Autodesk Inventor part; units mm, degrees
ref_plane "YZ Plane" through (0, 0, 0) normal (1, 0, 0) x (0, 1, 0)
ref_plane "XZ Plane" through (0, 0, 0) normal (0, 1, 0) x (-1, 0, 0)
ref_plane "XY Plane" through (0, 0, 0) normal (0, 0, 1) x (1, 0, 0)
sketch "CONTOURS" plane through (0, 0, 0) normal (0, 0, 1) x (1, 0, 0)
  line L0 (2153.8888, 619.2359) -> (2163.4719, 633.117)
  arc A0 (2185.9832, 634.7957) -> (2163.4719, 633.117) centre (2175.4045, 624.8791) ccw
  line L1 (2185.9832, 634.7957) -> (2411.1355, 394.6117)
  arc A1 (2406.7717, 371.5944) -> (2411.1355, 394.6117) centre (2400.5567, 384.695) ccw
  line L2 (2406.7717, 371.5944) -> (2360.367, 349.5799)
  arc A2 (2360.367, 349.5799) -> (2354.7432, 326.1016) centre (2367.0105, 335.5759) ccw
  line L3 (2354.7432, 326.1016) -> (2420.766, 240.6152)
  arc A3 (991.9076, 405.3519) -> (2420.766, 240.6152) centre (1790.9625, 1056.9921) ccw
  line L4 (991.9076, 405.3519) -> (1516.221, 700.5434)
  arc A4 (1516.221, 700.5434) -> (2065.5544, 700.5434) centre (1790.8877, 1057.1243) ccw
  line L5 (2065.5544, 700.5434) -> (2128.8659, 618.5677)
  arc A5 (2128.8659, 618.5677) -> (2153.8888, 619.2359) centre (2141.1332, 628.042) ccw
sketch "HOLES" plane through (0, 0, 0) normal (0, 0, 1) x (1, 0, 0)
  arc A0 (1449.9335, 932.975) -> (1455.5442, 933.6958) centre (1452.3785, 936.1408) ccw
  line L0 (1449.9335, 932.975) -> (1421.4416, 954.9799)
  arc A1 (1420.7208, 960.5906) -> (1421.4416, 954.9799) centre (1423.8866, 958.1456) ccw
  line L1 (1420.7208, 960.5906) -> (1427.4445, 969.2965)
  arc A2 (1433.0553, 970.0172) -> (1427.4445, 969.2965) centre (1430.6103, 966.8515) ccw
  line L2 (1433.0553, 970.0172) -> (1461.5471, 948.0124)
  arc A3 (1462.2679, 942.4017) -> (1461.5471, 948.0124) centre (1459.1022, 944.8467) ccw
  line L3 (581.1233, 599.0223) -> (574.9213, 608.1072)
  arc A4 (574.9213, 608.1072) -> (569.3624, 609.1555) centre (571.6177, 605.8519) ccw
  line L4 (569.3624, 609.1555) -> (539.6301, 588.858)
  arc A5 (539.6301, 588.858) -> (538.5818, 583.2991) centre (541.8854, 585.5544) ccw
  line L5 (538.5818, 583.2991) -> (544.7838, 574.2142)
  arc A6 (544.7838, 574.2142) -> (550.3427, 573.1659) centre (548.0874, 576.4695) ccw
  line L6 (550.3427, 573.1659) -> (580.075, 593.4634)
  arc A7 (580.075, 593.4634) -> (581.1233, 599.0223) centre (577.8197, 596.767) ccw
  line L7 (1171.3736, 565.7512) -> (1178.0973, 574.4571)
  arc A8 (1178.0973, 574.4571) -> (1177.3765, 580.0678) centre (1174.9316, 576.9021) ccw
  line L8 (1177.3765, 580.0678) -> (1148.8847, 602.0727)
  arc A9 (1148.8847, 602.0727) -> (1143.2739, 601.3519) centre (1146.4397, 598.9069) ccw
  line L9 (1143.2739, 601.3519) -> (1136.5502, 592.646)
  arc A10 (1136.5502, 592.646) -> (1137.271, 587.0353) centre (1139.716, 590.201) ccw
  line L10 (1137.271, 587.0353) -> (1165.7629, 565.0304)
  arc A11 (1165.7629, 565.0304) -> (1171.3736, 565.7512) centre (1168.2079, 568.1962) ccw
  line L11 (312.7987, 992.0706) -> (319.0007, 982.9857)
  arc A12 (317.9524, 977.4269) -> (319.0007, 982.9857) centre (315.6972, 980.7305) ccw
  line L12 (317.9524, 977.4269) -> (288.2201, 957.1293)
  arc A13 (282.6613, 958.1776) -> (288.2201, 957.1293) centre (285.9648, 960.4329) ccw
  line L13 (282.6613, 958.1776) -> (276.4592, 967.2625)
  arc A14 (277.5075, 972.8214) -> (276.4592, 967.2625) centre (279.7628, 969.5178) ccw
  line L14 (277.5075, 972.8214) -> (307.2399, 993.1189)
  arc A15 (312.7987, 992.0706) -> (307.2399, 993.1189) centre (309.4951, 989.8153) ccw
  arc A16 (877.4586, 807.9096) -> (881.5741, 811.7907) centre (877.5758, 811.9079) ccw
  line L15 (881.5741, 811.7907) -> (887.6999, 1020.7009)
  arc A17 (887.6999, 1020.7009) -> (883.8189, 1024.8164) centre (883.7016, 1020.8181) ccw
  line L16 (883.8189, 1024.8164) -> (872.8236, 1025.1388)
  arc A18 (872.8236, 1025.1388) -> (868.7081, 1021.2578) centre (872.7064, 1021.1405) ccw
  line L17 (868.7081, 1021.2578) -> (862.5822, 812.3476)
  arc A19 (862.5822, 812.3476) -> (866.4633, 808.232) centre (866.5805, 812.2303) ccw
  line L18 (866.4633, 808.232) -> (877.4586, 807.9096)
  arc A20 (370.076, 874.2818) -> (369.0277, 868.7229) centre (372.3312, 870.9782) ccw
  line L19 (369.0277, 868.7229) -> (486.8661, 696.1104)
  arc A21 (486.8661, 696.1104) -> (492.425, 695.062) centre (490.1697, 698.3656) ccw
  line L20 (492.425, 695.062) -> (501.5098, 701.2641)
  arc A22 (501.5098, 701.2641) -> (502.5581, 706.8229) centre (499.2546, 704.5677) ccw
  line L21 (502.5581, 706.8229) -> (384.7197, 879.4355)
  arc A23 (384.7197, 879.4355) -> (379.1608, 880.4838) centre (381.4161, 877.1802) ccw
  line L22 (379.1608, 880.4838) -> (370.076, 874.2818)
  line L23 (1833.6661, 426.4523) -> (1844.634, 427.2924)
  arc A24 (1833.6661, 426.4523) -> (1829.9832, 422.1586) centre (1833.9716, 422.464) ccw
  line L24 (1845.9439, 213.7689) -> (1829.9832, 422.1586)
  arc A25 (1101.2975, 659.9143) -> (1095.6868, 659.1936) centre (1098.8525, 656.7486) ccw
  arc A26 (1845.9439, 213.7689) -> (1850.2377, 210.086) centre (1849.9322, 214.0744) ccw
  arc A27 (2077.5111, 618.774) -> (2071.8727, 619.2297) centre (2074.4641, 616.1826) ccw
  line L25 (620.0838, 641.0058) -> (644.8608, 657.9204)
  arc A28 (644.8608, 657.9204) -> (645.9091, 663.4793) centre (642.6055, 661.224) ccw
  line L26 (645.9091, 663.4793) -> (639.707, 672.5642)
  arc A29 (639.707, 672.5642) -> (634.1482, 673.6125) centre (636.4035, 670.3089) ccw
  line L27 (634.1482, 673.6125) -> (609.3712, 656.6979)
  arc A30 (609.3712, 656.6979) -> (608.3229, 651.139) centre (611.6265, 653.3943) ccw
  line L28 (608.3229, 651.139) -> (614.525, 642.0541)
  arc A31 (614.525, 642.0541) -> (620.0838, 641.0058) centre (617.8286, 644.3094) ccw
  line L29 (1089.6839, 644.877) -> (1113.4271, 626.5396)
  arc A32 (1113.4271, 626.5396) -> (1119.0379, 627.2604) centre (1115.8721, 629.7054) ccw
  line L30 (1119.0379, 627.2604) -> (1125.7616, 635.9662)
  arc A33 (1125.7616, 635.9662) -> (1125.0408, 641.577) centre (1122.5958, 638.4112) ccw
  line L31 (1125.0408, 641.577) -> (1101.2975, 659.9143)
  arc A34 (1553.2327, 613.0929) -> (1551.9237, 618.5962) centre (1549.8265, 615.19) ccw
  line L32 (1095.6868, 659.1936) -> (1088.9631, 650.4877)
  arc A35 (1088.9631, 650.4877) -> (1089.6839, 644.877) centre (1092.1288, 648.0427) ccw
  line L33 (1266.2545, 230.909) -> (1272.0216, 240.2759)
  arc A36 (1277.5249, 241.5849) -> (1272.0216, 240.2759) centre (1275.4278, 238.1788) ccw
  line L34 (1277.5249, 241.5849) -> (1308.1804, 222.7106)
  arc A37 (1309.4894, 217.2073) -> (1308.1804, 222.7106) centre (1306.0833, 219.3045) ccw
  line L35 (1309.4894, 217.2073) -> (1303.7223, 207.8403)
  arc A38 (1298.219, 206.5313) -> (1303.7223, 207.8403) centre (1300.3161, 209.9375) ccw
  line L36 (1298.219, 206.5313) -> (1267.5635, 225.4056)
  arc A39 (1266.2545, 230.909) -> (1267.5635, 225.4056) centre (1269.6606, 228.8118) ccw
  line L37 (1515.7649, 636.1615) -> (1509.9977, 626.7945)
  arc A40 (1509.9977, 626.7945) -> (1511.3067, 621.2912) centre (1513.4039, 624.6974) ccw
  line L38 (1511.3067, 621.2912) -> (1541.9622, 602.4169)
  arc A41 (1541.9622, 602.4169) -> (1547.4655, 603.7259) centre (1544.0594, 605.8231) ccw
  line L39 (1547.4655, 603.7259) -> (1553.2327, 613.0929)
  line L40 (1551.9237, 618.5962) -> (1521.2682, 637.4705)
  arc A42 (1521.2682, 637.4705) -> (1515.7649, 636.1615) centre (1519.171, 634.0643) ccw
  line L41 (2048.564, 594.1557) -> (2055.6903, 585.7762)
  arc A43 (2055.6903, 585.7762) -> (2061.3288, 585.3206) centre (2058.7374, 588.3676) ccw
  line L42 (2061.3288, 585.3206) -> (2084.1818, 604.7561)
  arc A44 (2084.1818, 604.7561) -> (2084.6375, 610.3946) centre (2081.5904, 607.8032) ccw
  line L43 (2084.6375, 610.3946) -> (2077.5111, 618.774)
  line L44 (2071.8727, 619.2297) -> (2049.0196, 599.7942)
  arc A45 (2049.0196, 599.7942) -> (2048.564, 594.1557) centre (2051.611, 596.7471) ccw
  arc A46 (2196.184, 571.948) -> (2195.7283, 566.3095) centre (2198.7754, 568.9009) ccw
  line L45 (2195.7283, 566.3095) -> (2331.1291, 407.1002)
  arc A47 (2331.1291, 407.1002) -> (2336.7676, 406.6445) centre (2334.1762, 409.6916) ccw
  line L46 (2336.7676, 406.6445) -> (2345.147, 413.7708)
  arc A48 (2345.147, 413.7708) -> (2345.6027, 419.4093) centre (2342.5556, 416.8179) ccw
  line L47 (2345.6027, 419.4093) -> (2210.2019, 578.6187)
  arc A49 (2210.2019, 578.6187) -> (2204.5634, 579.0743) centre (2207.1548, 576.0273) ccw
  line L48 (2204.5634, 579.0743) -> (2196.184, 571.948)
  arc A50 (1339.7556, 342.3599) -> (1341.0646, 336.8566) centre (1343.1618, 340.2628) ccw
  line L49 (1339.7556, 342.3599) -> (1449.3315, 520.3322)
  arc A51 (1454.8349, 521.6412) -> (1449.3315, 520.3322) centre (1452.7377, 518.235) ccw
  line L50 (1454.8349, 521.6412) -> (1464.2018, 515.874)
  arc A52 (1465.5108, 510.3707) -> (1464.2018, 515.874) centre (1462.1047, 512.4678) ccw
  line L51 (1465.5108, 510.3707) -> (1355.9349, 332.3985)
  arc A53 (1350.4316, 331.0895) -> (1355.9349, 332.3985) centre (1352.5287, 334.4956) ccw
  line L52 (1350.4316, 331.0895) -> (1341.0646, 336.8566)
  line L53 (1462.2679, 942.4017) -> (1455.5442, 933.6958)
  arc A54 (1606.7292, 560.351) -> (1605.4201, 565.8543) centre (1603.323, 562.4481) ccw
  line L54 (1579.8739, 581.5829) -> (1605.4201, 565.8543)
  arc A55 (1579.8739, 581.5829) -> (1574.3706, 580.2739) centre (1577.7767, 578.1767) ccw
  line L55 (1568.6034, 570.9069) -> (1574.3706, 580.2739)
  arc A56 (1568.6034, 570.9069) -> (1569.9124, 565.4036) centre (1572.0096, 568.8098) ccw
  line L56 (1595.4587, 549.675) -> (1569.9124, 565.4036)
  arc A57 (1595.4587, 549.675) -> (1600.962, 550.984) centre (1597.5558, 553.0812) ccw
  line L57 (1606.7292, 560.351) -> (1600.962, 550.984)
  line L58 (1861.2056, 210.9261) -> (1850.2377, 210.086)
  arc A58 (1861.2056, 210.9261) -> (1864.8884, 215.2199) centre (1860.9001, 214.9144) ccw
  line L59 (1848.9278, 423.6095) -> (1864.8884, 215.2199)
  arc A59 (1848.9278, 423.6095) -> (1844.634, 427.2924) centre (1844.9394, 423.3041) ccw
  dimension "d13" = 122.5342
  dimension "d15" = 116.3458
  dimension "d17" = 116.3234
  dimension "d19" = 19
  dimension "d21" = 122.5114
  dimension "d23" = 30
  dimension "d25" = 36
  dimension "d27" = 36
  dimension "d29" = 29
sketch "LETTERS" plane through (0, 0, 0) normal (0, 0, 1) x (1, 0, 0)
  line L0 (1512.6274, 378.3219) -> (1504.8915, 360.2317)
  line L1 (1504.8915, 360.2317) -> (1513.0744, 356.7244)
  arc A0 (1517.2734, 366.5323) -> (1520.8186, 374.8004) centre (1519.042, 370.668) ccw
  line L2 (1517.2734, 366.5323) -> (1509.1534, 370.0046)
  arc A1 (1513.0744, 356.7244) -> (1517.2734, 366.5323) centre (1515.1759, 361.6275) ccw
  line L3 (1520.8186, 374.8004) -> (1512.6274, 378.3219)
extrude "Extrusion2" add sketch "CONTOURS" along normal blind 18
extrude "Extrusion3" cut sketch "HOLES" along normal blind 18 contours L23 A59 L59 A58 L58 A26 L24 A24 | L43 A44 L42 A43 L41 A45 L44 A27 | L39 A41 L38 A40 L37 A42 L40 A34 | L33 A36 L34 A37 L35 A38 L36 A39 | L48 A49 L47 A48 L46 A47 L45 A46 | L49 A51 L50 A52 L51 A53 L52 A50 | L57 A57 L56 A56 L55 A55 L54 A54
properties part number "Platform B1" material "Wood (Birch)"
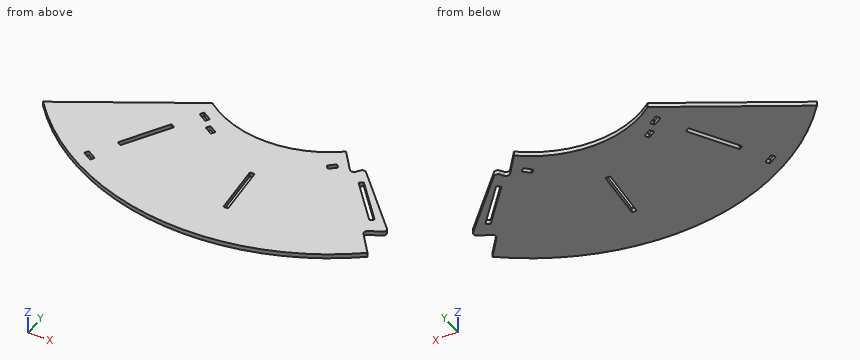
Here's how the part is built. I have some questions about the finished solid (model axes, mm). Round coordinates to 2 decimals unless told otherwise and drop trailing zeros. Order: outer loops, then holes, each group sorted by start corner. A loop starts at its lowest first (then second) coordinate and runs counter-clockwise, first axis right, second up. Notation, with made-up numbers: (19.5, 26) -> (36.5, 26) arc R16 cw to (36.5, 32) -> close; hole circle Ø6 at (48, 19.25). An arc over 180 degrees is marked (long way). Use a Markdown table: item, result. Add a question column.
(1) Suppose I cut it at C-C, the plane z = 9. Count the separate pieces of the cut face and the enclosed holes in it, and give its area (3 significant figures).
(2) Suppose I cut it at D-D, the plane x = 1150. Please give me the cut outline in (y, z), and give its area (3 significant figures).
(3) Suppose I cut it at B-B, the plane x = 1404.5. Please give me the cut outline in (y, z), and give its area (3 significant figures).
(4) I need wall thicknesses on line 1 along X through (y, z) = (364, 4.25); line 2 along X through (y, z) = (375, 7.5); line 3 along X through (y, z) = (267.5, 8.75). Which ranges of each line are inside material? Lowest first, please.
(5) For pin 1 Ø4 at (y, z) = (595, 13.5) entering from -X; pin 2 Ø1 at (x, z) = (2200, 7.5) entering from +Y; pin 3 Ø5 at (x, z) = (1750.5, 2) entering from +Y, each with a flat end and sliding along its axis, tell me the tip position at first contact or that it passes through.
(6) Suppose I cut it at A-A, the plane y = 456. Please give me the cut outline in (x, z).
Verdict:
| question | item | result |
|---|---|---|
| 1 | separate pieces | 1 |
| 1 | enclosed holes | 7 |
| 1 | area | 644,000 mm2 |
| 2 | outline | (249.35, 0) -> (494.36, 0) -> (494.36, 18) -> (249.35, 18) -> close |
| 2 | area | 4,410 mm2 |
| 3 | outline | (101.08, 0) -> (411.28, 0) -> (411.28, 18) -> (101.08, 18) -> close; (447.52, 0) -> (637.64, 0) -> (637.64, 18) -> (447.52, 18) -> close |
| 3 | area | 9,010 mm2 |
| 4 | line 1 | 1027.49 to 1353.08, 1375.39 to 1834.44, 1853.49 to 2390.76 |
| 4 | line 2 | 1017.65 to 1359.85, 1382.16 to 1833.6, 1852.65 to 2411.34 |
| 4 | line 3 | 1127.77 to 1841.83, 1860.88 to 2400 |
| 5 | pin 1 | x = 1325.2 |
| 5 | pin 2 | y = 620.38 |
| 5 | pin 3 | y = 609.07 |
| 6 | outline | (1081.87, 0) -> (1409.72, 0) -> (1409.72, 18) -> (1081.87, 18) -> close; (1432.04, 0) -> (2289.54, 0) -> (2289.54, 18) -> (1432.04, 18) -> close; (2314.48, 0) -> (2353.59, 0) -> (2353.59, 18) -> (2314.48, 18) -> close |
